Model file for the job. Use its own axes, mm. Round coordinates to 2 decimals unless told otherwise and drop trailing zeros. Order: outer loops, then holes, each group sorted by start corner. A loop starts at its lowest first (then second) coordinate and runs counter-clockwise, first axis right, second up. Notation, with made-up numbers: M -10.5,-38.75 L -2.5,-38.75 A11 ccw -2.5,-34.75 Z; hole C 38,35 d11. An arc over 180 degrees is marked long. Return JSON: item names as keys, results as strings. Group by question number.
Item 1: Probe line 1 along X through (y, z) = (0, 6) (3 decimals); line 2 along Y through (x, z) = (3, 5.75); line 3 along Y through (x, z) = (13, 3.75). List the from-to ranges inside material, lowest first.
Item 2: Slice it at A-A on x = 1.5. Write the cut outline in (y, z).
Item 3: Slice it at C-C on z = 3.5. Write the cut outline in (x, y) (3 decimals).
Item 4: Slice it at B-B on y = -7.5. Write the cut outline in (x, z) (3 decimals).
Item 5: Pin check, flat tip, straight feed: pin 1 Ø4 at (x, y) = (-11.91, -21.43) entering from -Z. Stop position of the tip, or through.
Item 6: Slice it at D-D on y = -22. Give the number of separate pieces and of enclosed holes in the cut face, then the cut area to 3 significant figures.
from build123d import *

# Parameters (mm, degrees)
SKETCH1_W                                         = 31.75
SKETCH1_H                                         = 50.8
BOSS_EXTRUDE1_DEPTH                               = 6.35
CUT_EXTRUDE2_DASH_027_DEPTH                       = 1.3208
CSK_FOR_4_FLAT_HEAD_MACHINE_SCREW_100_D           = 3.2639
CSK_FOR_4_FLAT_HEAD_MACHINE_SCREW_100_CSINK_D     = 5.715
CSK_FOR_4_FLAT_HEAD_MACHINE_SCREW_100_CSINK_ANGLE = 100


with BuildPart() as part:
    # Sketch1 → Boss-Extrude1 (new body)
    with BuildSketch(Plane.XY):
        Rectangle(SKETCH1_W, SKETCH1_H)
    extrude(amount=BOSS_EXTRUDE1_DEPTH)

    # Sketch3 → Cut-Extrude2 - dash 027 (cut)
    with BuildSketch(Plane.XY.offset(6.35)):
        with BuildLine():
            Line((13.3477, -11.176), (13.3477, 11.176))
            ThreePointArc((13.3477, 11.176), (10.848032113, 17.210732113), (4.8133, 19.7104))
            Line((4.8133, 19.7104), (-4.8133, 19.7104))
            ThreePointArc((-4.8133, 19.7104), (-10.848032113, 17.210732113), (-13.3477, 11.176))
            Line((-13.3477, 11.176), (-13.3477, -11.176))
            ThreePointArc((-13.3477, -11.176), (-10.848032113, -17.210732113), (-4.8133, -19.7104))
            Line((-4.8133, -19.7104), (4.8133, -19.7104))
            ThreePointArc((4.8133, -19.7104), (10.848032113, -17.210732113), (13.3477, -11.176))
        make_face()
        with BuildLine():
            Line((-4.8133, -17.526), (4.8133, -17.526))
            ThreePointArc((4.8133, -17.526), (9.303428061, -15.666128061), (11.1633, -11.176))
            Line((11.1633, -11.176), (11.1633, 11.176))
            ThreePointArc((11.1633, 11.176), (9.303428061, 15.666128061), (4.8133, 17.526))
            Line((4.8133, 17.526), (-4.8133, 17.526))
            ThreePointArc((-4.8133, 17.526), (-9.303428061, 15.666128061), (-11.1633, 11.176))
            Line((-11.1633, 11.176), (-11.1633, -11.176))
            ThreePointArc((-11.1633, -11.176), (-9.303428061, -15.666128061), (-4.8133, -17.526))
        make_face(mode=Mode.SUBTRACT)
    extrude(amount=-CUT_EXTRUDE2_DASH_027_DEPTH, mode=Mode.SUBTRACT)

    # CSK for #4 Flat Head Machine Screw (100)1 (through all)
    with Locations(Plane(origin=(0, 0, 0), x_dir=(-1, 0, 0), z_dir=(0, 0, -1))):
        with Locations((-11.90625, 21.43125), (11.90625, 21.43125), (-11.90625, -21.43125), (11.90625, -21.43125)):
            CounterSinkHole(CSK_FOR_4_FLAT_HEAD_MACHINE_SCREW_100_D / 2, CSK_FOR_4_FLAT_HEAD_MACHINE_SCREW_100_CSINK_D / 2, counter_sink_angle=CSK_FOR_4_FLAT_HEAD_MACHINE_SCREW_100_CSINK_ANGLE)


solid = part.part
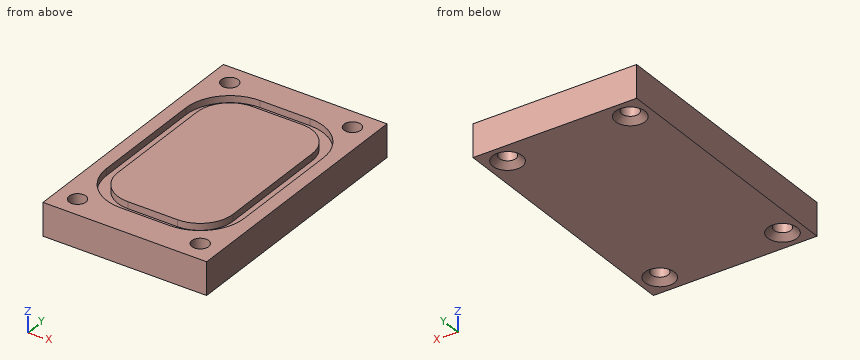
Output values:
{
 "1": {"line 1": "-15.875 to -13.348, -11.163 to 11.163, 13.348 to 15.875", "line 2": "-25.4 to -19.71, -17.53 to 17.53, 19.71 to 25.4", "line 3": "-25.4 to -22.64, -20.22 to 20.22, 22.64 to 25.4"},
 "2": {"outline": "M -25.4,0 L 25.4,0 L 25.4,6.35 L 19.71,6.35 L 19.71,5.03 L 17.53,5.03 L 17.53,6.35 L -17.53,6.35 L -17.53,5.03 L -19.71,5.03 L -19.71,6.35 L -25.4,6.35 Z"},
 "3": {"outline": "M -15.875,-25.4 L 15.875,-25.4 L 15.875,25.4 L -15.875,25.4 Z; hole C -11.906,-21.431 d3.264; hole C -11.906,21.431 d3.264; hole C 11.906,-21.431 d3.264; hole C 11.906,21.431 d3.264"},
 "4": {"outline": "M -15.875,0 L 15.875,0 L 15.875,6.35 L 13.348,6.35 L 13.348,5.029 L 11.163,5.029 L 11.163,6.35 L -11.163,6.35 L -11.163,5.029 L -13.348,5.029 L -13.348,6.35 L -15.875,6.35 Z"},
 "5": {"pin 1": "z = 0.72"},
 "6": {"separate pieces": "3", "enclosed holes": "0", "area": "160 mm²"}
}
